Work out the finished part from the listing and answer in its coordinate system (mm). A direction names the side the tool comes from. Give positions to 0.01 mm unless a question says otherwise; leave off trailing zeros. Order: outer loops, then holes, each group sorted by start corner. A loop starts at its lowest first (then second) coordinate and runs counter-clockwise, first axis right, second up.
Autodesk Inventor part; units mm, degrees
ref_plane "Work Plane2" through (25.5745, -91.5066, 0) normal (0, 0, 1) x (1, 0, 0)
ref_plane "YZ Plane" through (0, 0, 0) normal (1, 0, 0) x (0, 1, 0)
ref_plane "XZ Plane" through (0, 0, 0) normal (0, 1, 0) x (-1, 0, 0)
ref_plane "Work Plane1" through (50, -100, 0) normal (0, 0, 1) x (1, 0, 0)
sketch "Sketch1" plane through (50, -100, 0) normal (0, 0, 1) x (1, 0, 0)
  line L0 (-9.1, 25) -> (-9.1, 17.5) construction
  line L1 (-9.1, 25) -> (-25, 25) construction
  line L2 (-25, 25) -> (-25, 9.1) construction
  line L3 (-17.5, 9.1) -> (-25, 9.1) construction
  line L4 (-17.5, 9.1) -> (-17.5, 15.5) construction
  arc A0 (-15.5, 17.5) -> (-17.5, 15.5) centre (-15.5, 15.5) ccw construction
  line L5 (-15.5, 17.5) -> (-9.1, 17.5) construction
  circle A1 centre (-20, 20) radius 2.2989 construction
  line L6 (-40.9, 17.5) -> (-40.9, 25)
  line L7 (-40.9, 17.5) -> (-34.5, 17.5) construction
  arc A2 (-32.5, 15.5) -> (-34.5, 17.5) centre (-34.5, 15.5) ccw construction
  line L8 (-32.5, 15.5) -> (-32.5, 9.1) construction
  line L9 (-25, 9.1) -> (-32.5, 9.1)
  line L10 (-25, 9.1) -> (-25, 25) construction
  line L11 (-25, 25) -> (-40.9, 25) construction
  circle A3 centre (-30, 20) radius 2.2989 construction
  line L12 (-40.9, 25) -> (-40.9, 32.5) construction
  line L13 (-40.9, 25) -> (-25, 25)
  line L14 (-25, 25) -> (-25, 40.9) construction
  line L15 (-32.5, 40.9) -> (-25, 40.9) construction
  line L16 (-32.5, 40.9) -> (-32.5, 34.5) construction
  arc A4 (-34.5, 32.5) -> (-32.5, 34.5) centre (-34.5, 34.5) ccw construction
  line L17 (-34.5, 32.5) -> (-40.9, 32.5) construction
  circle A5 centre (-30, 30) radius 2.2989 construction
  circle A6 centre (-20, 30) radius 2.2989 construction
  line L18 (-25, 40.9) -> (-17.5, 40.9) construction
  line L19 (-25, 40.9) -> (-25, 25) construction
  line L20 (-25, 25) -> (-9.1, 25) construction
  line L21 (-9.1, 32.5) -> (-9.1, 25) construction
  line L22 (-9.1, 32.5) -> (-15.5, 32.5) construction
  arc A7 (-17.5, 34.5) -> (-15.5, 32.5) centre (-15.5, 34.5) ccw construction
  line L23 (-17.5, 34.5) -> (-17.5, 40.9) construction
  line L24 (-25, 9.1) -> (-32.5, 9.1)
  line L25 (-40.9, 17.5) -> (-32.5, 9.1)
  line L26 (-40.9, 17.5) -> (-40.9, 25)
  line L27 (-25, 25) -> (-40.9, 25)
  line L28 (-25, 9.1) -> (-25, 25)
  arc A8 (-32.5755, 19.3934) -> (-26.2755, 19.3934) centre (-29.4255, 19.3934) ccw
  circle A9 centre (-29.4255, 19.3934) radius 3.75
  line L29 (-40.9, 17.5) -> (-40.9, 25)
  line L30 (-25, 9.1) -> (-32.5, 9.1)
  line L31 (-40.9, 25) -> (-25, 25)
  point P0 (-50, 100)
  dimension "d0" = 7.5
extrude "Extrusion1" add sketch "Sketch1" along normal blind 1.5
sketch "Sketch2" plane through (50, -100, 0) normal (0, 0, -1) x (-1, 0, 0)
  circle A0 centre (29.4255, 19.3934) radius 3.75
  line L0 (25, 25) -> (40.9, 25)
  line L1 (25, 9.1) -> (25, 25)
  line L2 (32.5, 9.1) -> (25, 9.1)
  line L3 (40.9, 17.5) -> (32.5, 9.1)
  line L4 (40.9, 25) -> (40.9, 17.5)
  line L5 (32.5, -15.5) -> (32.5, 15.5)
  arc A1 (34.5, 17.5) -> (32.5, 15.5) centre (34.5, 15.5) ccw
  line L6 (34.5, 17.5) -> (65.5, 17.5)
  line L7 (65.9987, 17.7) -> (34.5, 17.7)
  arc A2 (34.5, 17.7) -> (32.3, 15.5) centre (34.5, 15.5) ccw
  line L8 (32.3, 15.5) -> (32.3, -15.5)
  line L9 (40.9, 17.5) -> (32.5, 9.1)
  point P0 (50, 100)
  point P1 (41.1, 17.7)
  point P2 (32.3, 8.9)
  dimension "d9" = 0.2
extrude "Extrusion2" add sketch "Sketch2" along normal blind 5 draft -3 contours L3 L5 A1 L6
pattern_circular "Circular Pattern1" count 2 over 90 about axis through (25, -75, 0) along (0, 0, 1) of "Extrusion1", "Extrusion2"
sketch "Sketch3" plane through (50, -100, 1.5) normal (0, 0, 1) x (1, 0, 0)
  circle A0 centre (-19.3934, 20.5745) radius 3.75
  circle A1 centre (-29.4255, 19.3934) radius 3.75
  line L0 (-9.1, 25) -> (-40.9, 25)
  line L1 (-40.9, 25) -> (-40.9, 17.5)
  line L2 (-40.9, 17.5) -> (-32.5, 9.1)
  line L3 (-32.5, 9.1) -> (-17.5, 9.1)
  line L4 (-17.5, 9.1) -> (-9.1, 17.5)
  line L5 (-9.1, 17.5) -> (-9.1, 25)
  line L6 (-40.9, 25) -> (-9.1, 25)
  line L7 (-9.1, 25) -> (-9.1, 28)
  line L8 (-9.1, 28) -> (-40.9, 28)
  line L9 (-40.9, 28) -> (-40.9, 25)
  point P0 (-50, 100)
  dimension "d10" = 3
ref_plane "Work Plane2" through (25.5745, -91.5066, 0) normal (0, 0, 1) x (1, 0, 0)
extrude "Extrusion3" add sketch "Sketch3" against normal up to surface (1.5 mm away) contours L0 L9 L8 L7
sketch "Sketch4" plane through (40.9, -82.5, 1.5) normal (1, 0, 0) x (0, 0, -1)
  line L0 (1.5, 6.8934) -> (9.5, 6.8934) construction
  line L1 (6.5, -7.7674) -> (6.5, -0.262)
  line L2 (1.5, 0) -> (1.5, 10.5) construction
  line L3 (1.5, 10.5) -> (6.5, 10.5) construction
  line L4 (0, 10.5) -> (1.5, 10.5)
  line L5 (1.5, 10.5) -> (6.5, 10.5)
  line L6 (1.5, 10.5) -> (1.5, 6.6716)
  line L7 (6.5, 10.5) -> (6.5, 7.1108) construction
  line L8 (6.5, 7.1108) -> (1.5, 6.8487)
  line L9 (1.5, 6.8487) -> (1.5, 10.5)
  line L10 (6.5, 10.5) -> (6.5, 7.1108)
  point P0 (1.5, 82.5)
  dimension "d16" = 93
extrude "Extrusion4" add sketch "Sketch4" against normal up to surface (31.2255 mm away)
properties part number "30_Baseplate_Connector_Clamp"
1. Which of the six approach directions +Z, -Z, +X, -X, +Y, -Y give full straight-line access (tool end or side, diameter ignored) to faces 4 (the face through (9.674, -74, -2)), 5 (the face through (25, -83, 0)), 6 (the face through (25.51, -75.52, -2.54)), 7 (the face through (17.37, -87.74, -2.47)), 8 (the face through (25, -90.9, 1))?
Findings below:
face 4: -Z, -X, +Y
face 5: -Z
face 6: -Z, +X, -X
face 7: -Z, -Y
face 8: +Z, -Z, +X, -X, -Y
2. The part is cut by section D-D (y = -88.75). Write down the section's boundary in (x, z).
Findings below:
outline: (15.35, 0) - (15.72, -5) - (17.24, -5) - (17.5, 0) - (32.5, 0) - (32.76, -5) - (34.28, -5) - (34.65, 0) - (34.65, 1.5) - (15.35, 1.5) - close
3. Straight lines are drawn through the part: probe 1 along X at (y, z) = (-78.75, 0.75); probe 2 along X at (y, z) = (-82.25, 1.25); probe 3 along X at (y, z) = (-73.5, -2.5). For each, find the intervals that lie inside material, in ascending order.
Findings below:
probe 1: x = 9.1 to 17.32, 23.83 to 26.92, 34.3 to 40.9
probe 2: x = 9.1 to 17.2, 23.95 to 28.14, 33.07 to 40.9
probe 3: x = 9.67 to 40.9
4. The mould has two halves that part along X. Classify faces 1 (the face through (13.2, -86.6, 0.7)), 2 (the face through (14, -86, -5)), 3 (the face through (33.14, -82.19, 0.74)): pulls with the +X half, pulls with the -X half, needs draft (parallel to the pull), parting line crosses it, or undercut.
Findings below:
face 1: pulls with the -X half
face 2: needs draft
face 3: undercut
5. The part is cut by section A-A (z = -1.25). Write down the section's boundary in (x, y).
Findings below:
outline: (9.26, -82.57) - (17.43, -90.74) - (17.43, -84.5) arc R1.93 ccw to (15.5, -82.57) - close; (9.67, -75.59) - (40.9, -75.59) - (40.9, -72) - (9.67, -72) - close; (32.57, -90.74) - (40.74, -82.57) - (34.5, -82.57) arc R1.93 ccw to (32.57, -84.5) - close
6. The part is cut by section B-B (y = -78). Write down the section's boundary in (x, z), then the cut area to 3 significant figures.
Findings below:
outline: (9.1, 0) - (17.88, 0) - (17.88, 1.5) - (9.1, 1.5) - close; (23.27, 0) - (27.14, 0) - (27.14, 1.5) - (23.27, 1.5) - close; (34.08, 0) - (40.9, 0) - (40.9, 1.5) - (34.08, 1.5) - close
area: 29.2 mm2
7. Given P1, Ø1.1, axis at y = -73.5, z = -3, coming from the -X side; P2, Ø7, axis at x = 30.61, y = -79.43, coming from the +Z side; P3, Ø1.5, axis at y = -85.5, z = 0, coming from the -X side; P4, Ø8.5, axis at x = 20.57, y = -80.61, coming from the -Z side, each flat-ended and moving along its own axis, determine where each tip first touches the part or whether it passes through.
Findings below:
P1: stops at x = 9.67
P2: passes through
P3: stops at x = 11.35
P4: stops at z = 0
8. The part is cut by section C-C (x = 31). Write down the section's boundary in (y, z), then the cut area to 3 significant figures.
Findings below:
outline: (-90.9, 0) - (-83.15, 0) - (-83.15, 1.5) - (-90.9, 1.5) - close; (-75.7, 0) - (-75.65, 0) - (-75.39, -5) - (-72, -5) - (-72, 1.5) - (-75.7, 1.5) - close
area: 34.8 mm2
